```python
from build123d import *

# Parameters (mm, degrees)
F2_DEPTH  = 25
F3_DEPTH  = 20
F6_DEPTH  = 50
F8_R      = 12.5
F9_DEPTH  = 54.4
F7_R      = 12.5
F10_DEPTH = 25


with BuildPart() as f2:
    # F0 (on Front) → F2 (new body, symmetric)
    with BuildSketch(Plane.XZ):
        Polygon((-43.145511, 0), (-20, 0), (20, 0), (43.145511, 0), (43.145511, 20), (20, 20), (20, 50), (-20, 50), (-20, 20), (-43.145511, 20), align=None)
    extrude(amount=F2_DEPTH, both=True)

    # F1 (on Top) → F3 (join)
    with BuildSketch(Plane.XY):
        with BuildLine():
            Line((-43.145511, -25), (-43.145511, 25))
            ThreePointArc((-43.145511, 25), (-68.145511, 0), (-43.145511, -25))
        make_face()
    extrude(amount=F3_DEPTH)

    # F4: F2 across plane


with BuildPart() as f2_1:
    add(f2.part)
    add(f2.part.mirror(Plane.YZ))

    # F5 (on face) → F6 (join)
    with BuildSketch(Plane.XZ.offset(25)):
        with BuildLine():
            Line((-20, 50), (20, 50))
            ThreePointArc((20, 50), (0, 70), (-20, 50))
        make_face()
    extrude(amount=-F6_DEPTH)

    # F8 (on face) → F9 (cut, symmetric)
    with BuildSketch(Plane(origin=(0, 25, 0), x_dir=(-1, 0, 0), z_dir=(0, 1, 0))):
        with Locations((0, 50)):
            Circle(F8_R)
    extrude(amount=F9_DEPTH, both=True, mode=Mode.SUBTRACT)

    # F7 (on face) → F10 (cut)
    with BuildSketch(Plane.XY.offset(20)):
        with Locations((43.145511, 0)):
            Circle(F7_R)
        with Locations((-43.145511, 0)):
            Circle(F7_R)
    extrude(amount=-F10_DEPTH, mode=Mode.SUBTRACT)


solid = f2_1.part
```
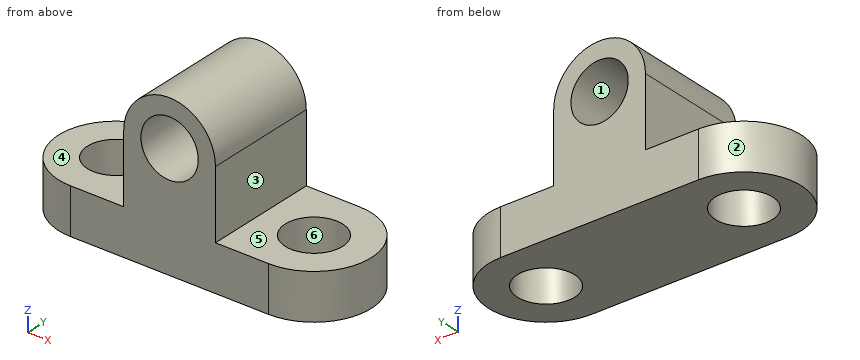
Check sheet for the modelled part. Datum: model origin and axes. Units: mm. Face numbers are marked on the shaded views. A direction names the side the tool comes from. Round coordinates to 2 decimals unless told otherwise and drop trailing zeros. Loops run counter-clockwise (first coordinate to the right, second up) from the corner with the lowest first, then second, coordinate; pieces in that order, holes last. Notation, with made-up numbers: (3, 59) - (52, 59) arc R25 cw to (52, 76) - close; hole circle Ø2 at (36, 77). An arc over 180 degrees is marked (long way). Answer as a JSON object with one key per item and string values. Group by question number.
Q1. Set-up check for the marked faces 4, 5 and 6: record each of +Z, -Z, +X, -X, +Y, -Y from which the full face is reachable in a straight line by a thin tool's end or side.
Q2. Sectioned sample at C-C, the plane z = 17.5. Enter the section's corners in (x, y), plus the area to 3 significant figures.
Q3. Sectioned sample at A-A, the plane y = 0. Enter the section's corners in (x, z).
Q4. Scan lines: line 1 along Z through (x, y) = (0, 7); line 2 along X through (y, z) = (-2, 23); line 3 along Z through (x, y) = (35, -16). Record each from-to range of solid material in increasing order. Write a range as [from, to].
Q5. Gauge pin test, flat ends, axial feed: P1, Ø22.5, axis at x = 43.15, y = 0, coming from the -Z side; P2, Ø12, axis at x = 23, y = 9, coming from the +Z side; P3, Ø5, axis at y = -3, z = 57, coming from the +X side; P4, Ø24, axis at y = 8, z = 37.5, coming from the +X side. Record the tip position at first contact, or that the pin passes through.
Q6. Mould release check, pull along X, two halves, no side actions. Record for the marked faces 1, 2 and 3: released by +X, released by -X, zero draft, split by the parting line, or undercut.
Q7. Sectioned sample at B-B, the plane x = 0. Enter the section's corners in (y, z), plus the area to 3 significant figures.
Q8. Sectioned sample at D-D, the plane z = 56.5. Enter the section's corners in (x, y), plus the area to 3 significant figures.
Solution:
{
 "1": {"face 4": "+Z, -X, +Y, -Y", "face 5": "+Z, +X, +Y, -Y", "face 6": "+Z, -Z"},
 "2": {"outline": "(-43.15, -25) - (43.15, -25) arc R25 ccw to (43.15, 25) - (-43.15, 25) arc R25 ccw to start; hole circle Ø25 at (-43.15, 0); hole circle Ø25 at (43.15, 0)", "area": "5,300 mm²"},
 "3": {"outline": "(-68.15, 0) - (-55.65, 0) - (-55.65, 20) - (-68.15, 20) - close; (-30.65, 0) - (30.65, 0) - (30.65, 20) - (20, 20) - (20, 50) arc R20 ccw to (-20, 50) - (-20, 20) - (-30.65, 20) - close; (55.65, 0) - (68.15, 0) - (68.15, 20) - (55.65, 20) - close; hole circle Ø25 at (0, 50)"},
 "4": {"line 1": "z = [0, 37.5], [62.5, 70]", "line 2": "x = [-20, 20]", "line 3": "z = [0, 20]"},
 "5": {"P1": "passes through", "P2": "stops at z = 60.54", "P3": "stops at x = 19.49", "P4": "stops at x = 20"},
 "6": {"face 1": "undercut", "face 2": "released by -X", "face 3": "released by +X"},
 "7": {"outline": "(-25, 0) - (25, 0) - (25, 37.5) - (-25, 37.5) - close; (-25, 62.5) - (25, 62.5) - (25, 70) - (-25, 70) - close", "area": "2,250 mm²"},
 "8": {"outline": "(-18.91, -25) - (-10.68, -25) - (-10.68, 25) - (-18.91, 25) - close; (10.68, -25) - (18.91, -25) - (18.91, 25) - (10.68, 25) - close", "area": "824 mm²"}
}
